Check sheet for the modelled part. Datum: model origin and axes. Units: mm. A direction names the side the tool comes from. Give positions to 0.01 mm unless a question says otherwise; leave off trailing zeros. Order: outer loops, then holes, each group sorted by start corner. A loop starts at its lowest first (then second) coordinate and runs counter-clockwise, first axis right, second up. Notation, with made-up numbers: (-17.5, 42) - (20.5, 42) arc R32 cw to (20.5, 80) - close; hole circle Ø11 at (-9, 83). An arc over 180 degrees is marked (long way). Answer in a Markdown table with one row per item.
from build123d import *

# Parameters (mm, degrees)
SKETCH3_R           = 1.65
BOSS_EXTRUDE1_DEPTH = 3
BOSS_EXTRUDE2_DEPTH = 5
SKETCH11_W          = 2.655817679
SKETCH11_H          = 5
BOSS_EXTRUDE6_DEPTH = 6
SKETCH12_W          = 5
SKETCH12_H          = 1.502128234
BOSS_EXTRUDE7_DEPTH = 5
SKETCH13_R          = 1.5
CUT_EXTRUDE3_DEPTH  = 5


with BuildPart() as part:
    # Sketch3 → Boss-Extrude1 (new body)
    with BuildSketch(Plane.XY):
        with BuildLine():
            Line((-4, 0), (-4, 15))
            ThreePointArc((-4, 15), (0, 19), (4, 15))
            Line((4, 15), (4, 0))
            ThreePointArc((4, 0), (0, -4), (-4, 0))
        make_face()
        Circle(SKETCH3_R, mode=Mode.SUBTRACT)
    extrude(amount=BOSS_EXTRUDE1_DEPTH)

    # Sketch4 → Boss-Extrude2 (add)
    with BuildSketch(Plane.XY.offset(3)):
        with BuildLine():
            Line((0, 16), (20, 16))
            ThreePointArc((20, 16), (21, 15), (20, 14))
            Line((20, 14), (0, 14))
            ThreePointArc((0, 14), (-1, 15), (0, 16))
        make_face()
    extrude(amount=BOSS_EXTRUDE2_DEPTH)

    # Sketch11 → Boss-Extrude6 (add)
    with BuildSketch(Plane.XZ.offset(-14)):
        with Locations((18.672091161, 5.5)):
            Rectangle(SKETCH11_W, SKETCH11_H)
    extrude(amount=BOSS_EXTRUDE6_DEPTH)

    # Sketch12 → Boss-Extrude7 (add)
    with BuildSketch(Plane(origin=(20, 0, 0), x_dir=(0, 0, -1), z_dir=(1, 0, 0))):
        with Locations((-5.5, 8.751064117)):
            Rectangle(SKETCH12_W, SKETCH12_H)
    extrude(amount=BOSS_EXTRUDE7_DEPTH)

    # Sketch13 → Cut-Extrude3 (cut)
    with BuildSketch(Plane(origin=(0, 9.502128234, 0), x_dir=(1, 0, 0), z_dir=(0, 1, 0))):
        with Locations(Location((22.5, -5.5, 0), (0, 0, 270))):
            Circle(SKETCH13_R)
    extrude(amount=-CUT_EXTRUDE3_DEPTH, mode=Mode.SUBTRACT)


solid = part.part
(1) Thickness scan on L1, parallel to X at y = 8.95, z = 5.5; L2, parallel to Y at x = 0, z = 1.7; L3, parallel to Z at x = -2, y = 1.25. Record the ranges inside material, lowest first.
Geometry says:
| item | result |
|---|---|
| L1 | 17.34 to 21, 24 to 25 |
| L2 | -4 to -1.65, 1.65 to 19 |
| L3 | 0 to 3 |
(2) Mould release check, pull along Z, two halves, no side actions. Record for faces 4 (the flat face through (16, 14.4, 3)), 5 (the cylindrical face through (23.987, 8.762, 5.305)), 6 (the cylindrical face through (-1, 15, 5)): pulls with the +Z half, pulls with the -Z half, needs draft (parallel to the pull), parting line crosses it, or undercut.
Geometry says:
| item | result |
|---|---|
| face 4 | pulls with the -Z half |
| face 5 | undercut |
| face 6 | needs draft |
(3) Cross-section at C-C, the plane x = 2.5. Record the cut outline in (y, z).
Geometry says:
| item | result |
|---|---|
| outline | (-3.12, 0) - (18.12, 0) - (18.12, 3) - (16, 3) - (16, 8) - (14, 8) - (14, 3) - (-3.12, 3) - close |
(4) Cross-section at D-D, the plane x = -0.5. Record the cut outline in (y, z).
Geometry says:
| item | result |
|---|---|
| outline | (-3.97, 0) - (-1.57, 0) - (-1.57, 3) - (-3.97, 3) - close; (1.57, 0) - (18.97, 0) - (18.97, 3) - (15.87, 3) - (15.87, 8) - (14.13, 8) - (14.13, 3) - (1.57, 3) - close |
(5) Gauge pin test, flat ends, axial feed: P1, Ø4, axis at x = 9.5, z = 6.5, coming from the -Y side; P2, Ø2.5, axis at y = 4.5, z = 1, coming from the +X side; P3, Ø1.5, axis at x = 10, y = 15, coming from the -Z side; P4, Ø9, axis at x = -0.5, y = 11, coming from the +Z side. Record the tip position at first contact, or that the pin passes through.
Geometry says:
| item | result |
|---|---|
| P1 | y = 14 |
| P2 | x = 4 |
| P3 | z = 3 |
| P4 | z = 8 |
(6) Access from +Z, -Z, +X, -X, +Y, -Y to the whole of each face (thin tool, end or side, straight path). Record for faces 1 (the flat face through (9, 14, 5)), 2 (the flat face through (20, 12, 5)), 3 (the flat face through (17.344, 11, 5)).
Geometry says:
| item | result |
|---|---|
| face 1 | +Z, -X, -Y |
| face 2 | +Z, -Z, +X |
| face 3 | +Z, -Z, -X, -Y |
(7) Cross-section at B-B, the plane x = 23. Record the cut outline in (y, z).
Geometry says:
| item | result |
|---|---|
| outline | (8, 3) - (9.5, 3) - (9.5, 4.09) - (8, 4.09) - close; (8, 6.91) - (9.5, 6.91) - (9.5, 8) - (8, 8) - close |
(8) Cross-section at A-A, the plane z = 6.5. Record the cut outline in (x, y), then the cut area to 3 significant figures.
Geometry says:
| item | result |
|---|---|
| outline | (0, 14) - (17.34, 14) - (17.34, 8) - (21.38, 8) - (21.38, 9.5) - (20, 9.5) - (20, 14) arc R1 ccw to (20, 16) - (0, 16) arc R1 ccw to start; (23.62, 8) - (25, 8) - (25, 9.5) - (23.62, 9.5) - close |
| area | 63.2 mm² |
